from build123d import *

# Parameters (mm, degrees)
F1_DEPTH = 18.9992
F3_D     = 19.05
F4_D     = 12.7
F5_R     = 4.3873111452
F6_DEPTH = 25.4
F7_SIZE  = 1.27


with BuildPart() as f1:
    # F0 (on Front) → F1 (new body)
    with BuildSketch(Plane.XZ):
        Polygon((-52.6177957654, 0), (-52.6177957654, -60.96), (-1.8177957654, -60.96), (-1.8177957654, 0), (-14.5472735167, 32.9634994268), (-34.6658416092, 32.9634994268), (-42.0942343771, 32.9634994268), align=None)
    extrude(amount=F1_DEPTH)

    # F3 (through all)
    with Locations(Plane.XZ.offset(18.9992)):
        with Locations((-29.7135785222, 15.9400962293)):
            Hole(F3_D / 2)

    # F4 (through all)
    with Locations(Plane.XZ.offset(18.9992)):
        with Locations((-29.4040627778, -45.3441590071)):
            Hole(F4_D / 2)

    # F5 (on face) → F6 (cut)
    with BuildSketch(Plane.XY.offset(32.9634994268)):
        with Locations((-26.6399271786, -8.7757343426)):
            Circle(F5_R)
    extrude(amount=-F6_DEPTH, mode=Mode.SUBTRACT)

    # F7
    f7_edges = [f1.edges().sort_by_distance(p)[0] for p in [
        (-47.356015, 0, 16.48175),
        (-52.617796, 0, -30.48),
        (-1.817796, 0, -30.48),
        (-8.182535, 0, 16.48175),
        (-28.320754, 0, 32.963499),
        (-35.754063, -18.9992, -45.344159),
        (-39.238579, -18.9992, 15.940096),
        (-39.238579, 0, 15.940096),
        (-35.754063, 0, -45.344159),
    ]]
    chamfer(f7_edges, length=F7_SIZE)


solid = f1.part
Source: CAD feature listing. Evaluate the final solid. Frame: model axes, mm. A direction names the side the tool comes from. Give positions to 0.01 mm unless a question says otherwise; leave off trailing zeros. Write each loop counter-clockwise with the first axis right and the second up, starting at its lowest first coordinate (ties: lowest second). Pieces come first, ordered by that corner, then holes. Notation, with made-up numbers: (77.5, 16) - (99.5, 16) arc R7 cw to (99.5, 29) - close; hole circle Ø5 at (43, 47). An arc over 180 degrees is marked (long way). Write item = value, one per line. Start each with the question number.
Q1. Pin query (flat end, axial travel): pin 1 Ø1.5 at (x, y) = (-23.5, -7) entering from +Z; pin 2 Ø2 at (y, z) = (-6.5, 20) entering from +X (3 decimals); pin 3 Ø10 at (y, z) = (-15.5, 15.5) entering from -X. Return the tip coordinate at first contact, or that it passes through.
Q2. Material intervals for probe 1 along Z at (x, y) = (-24, -6); probe 2 along X at (y, z) = (-7.75, 16); probe 3 along Z at (x, y) = (-37.5, -16.75), sorted ascending.
Q3. Draft query along Z for faces 1 (the cylindrical face through (-35.46, -9.38, -43.44)), 2 (the flat face through (-1.818, -10, -31)), 3 (the flat face through (-8.69, -0.63, 16.02)). Return one class per face: +Z half, -Z half, draft (parallel to the pull), parting line (faces both ways), or undercut.
Q4. Reachability of faces 4 (the cylindrical face through (-22.253, -8.851, 8.536)), 5 (the flat face through (-52.618, -10, -30)) from +Z, -Z, +X, -X, +Y, -Y: full face, straight path, thin tool, end or side. Return the list, or none.
Q5. Cut plane C-C, the plane x = -6.5. Return loops of the section in (y, z), then the cut area to 3 significant figures.
Q6. Cut plane B-B, the plane x = -12.5. Return loops of the section in (y, z).
Computed values:
q1.pin_1 = 7.56
q1.pin_2 = -9.155
q1.pin_3 = -49.27
q2.probe_1 = -60.96 to -48.68, -42.01 to 7.56
q2.probe_2 = -47.51 to -39.24, -20.19 to -8
q2.probe_3 = -60.96 to 10.45, 21.43 to 32.96
q3.face_1 = undercut
q3.face_2 = draft
q3.face_3 = +Z half
q4.face_4 = +Z
q4.face_5 = +Z, -Z, -X, +Y, -Y
q5.outline = (-19, -60.96) - (0, -60.96) - (0, 8.6) - (-1.27, 12.12) - (-19, 12.12) - close
q5.area = 1,390 mm²
q6.outline = (-19, -60.96) - (0, -60.96) - (0, 24.14) - (-1.27, 27.66) - (-19, 27.66) - close
